The listing builds one solid part. Answer for the finished solid, in the listing's coordinates (mm). Face numbers are marked on the shaded views. A direction names the side the tool comes from. Round coordinates to 2 decimals unless told otherwise and drop trailing zeros. Write each loop counter-clockwise with the first axis right and the second up, starting at its lowest first coordinate (ties: lowest second). Pieces come first, ordered by that corner, then holes.
Item 1: Find section C-C on y = -3.75. Give the vertices of the cut face in (x, z).
Item 2: Each of these flat-tipped pins is pushed along its axis until it touches: pin 1 (3.5 mm diameter, centred on y = -4, z = -0.5, fed in from -X); pin 2 (1.2 mm diameter, centred on x = -0.5, y = -6.5, fed in from -Z); pin 3 (2.5 mm diameter, centred on x = -1.8, z = -1.2, fed in from -Y); pin 4 (1.5 mm diameter, centred on x = -1.5, z = 0.5, fed in from +Y). Where does it stop, or does it pass through?
Item 3: Find section A-A on x = 1.65. Give the vertices of the cut face in (y, z), then the cut area to 3 significant figures.
Item 4: A tool of negligible diameter and unlimited length cuts with its end or side. For the marked faces 5, 6 and 7, from which of +Z, -Z, +X, -X, +Y, -Y can it reach the whole face along a straight path? Write none if from no direction.
Item 5: Find section D-D on x = -0.55. Give the vertices of the cut face in (y, z), then the cut area to 3 significant figures.
Item 6: Find the intervals of material crossed by probe 1 along Y at (x, z) = (1.1, 0); probe 2 along X at (y, z) = (-7.05, 2.3); probe 3 along X at (y, z) = (-0.25, -2.25), in increasing order.
Item 7: For a pull along Z with two mould halves and no side action, classify the marked faces 1, 2, 3 and 4 as +Z half, -Z half, draft (parallel to the pull), parting line (faces both ways), or undercut.
Item 8: Find section B-B on z = 0. Give the vertices of the cut face in (x, y), then the cut area to 3 significant figures.
```python
from build123d import *

# Parameters (mm, degrees)
SKETCH_1_R          = 1.4
EXTRUDE_1_DEPTH     = 2
SKETCH_2_W          = 5.2
SKETCH_2_H          = 7
SKETCH_2_R          = 0.8
EXTRUDE_2_DEPTH     = 1.5
SKETCH_5_W          = 6
SKETCH_5_H          = 1
CUT_EXTRUDE_1_DEPTH = 2.5
CUT_EXTRUDE_2_REACH = 12.163
FILLET_1_R          = 0.2
FILLET_2_R          = 0.2
CHAMFER_1_SIZE      = 0.2


with BuildPart() as part:
    # 草图1 → 凸台-拉伸1 (new body)
    with BuildSketch(Plane(origin=(0, 0, 0), x_dir=(0, 0, -1), z_dir=(1, 0, 0))):
        with BuildLine():
            Line((3.5, 0), (3.5, -8))
            Line((3.5, -8), (-3.5, -8))
            Line((-3.5, -8), (-3.5, 0))
            ThreePointArc((-3.5, 0), (0, 3.5), (3.5, 0))
        make_face()
        Circle(SKETCH_1_R, mode=Mode.SUBTRACT)
    extrude(amount=EXTRUDE_1_DEPTH)

    # 草图2 → 凸台-拉伸2 (add)
    with BuildSketch(Plane.XZ.offset(8)):
        with Locations((-0.6, 0)):
            Rectangle(SKETCH_2_W, SKETCH_2_H)
        with Locations(Location((-1.8, -1.2, 0), (0, 0, 270))):
            Circle(SKETCH_2_R, mode=Mode.SUBTRACT)
        with Locations(Location((-1.8, 2.3, 0), (0, 0, 270))):
            Circle(SKETCH_2_R, mode=Mode.SUBTRACT)
    extrude(amount=-EXTRUDE_2_DEPTH)

    # 草图5 → 切除-拉伸1 (cut)
    with BuildSketch(Plane.XZ.offset(8)):
        with Locations((-1, -3)):
            Rectangle(SKETCH_5_W, SKETCH_5_H)
    extrude(amount=-CUT_EXTRUDE_1_DEPTH, mode=Mode.SUBTRACT)

    # 草图6 → 切除-拉伸2 (cut, up to next)
    with BuildSketch(Plane.ZY.offset(3.2), mode=Mode.PRIVATE) as cut_extrude_2_sk1:
        with BuildLine():
            Line((-1, -8.325127743), (-3.27705392, -8.325127743))
            Line((-3.27705392, -8.325127743), (-3.27705392, -6))
            Line((-3.27705392, -6), (-2.897366596, -6))
            ThreePointArc((-2.897366596, -6), (-2.378404875, -7.407669683), (-1, -8))
            Line((-1, -8), (-1, -8.325127743))
        make_face()
    cut_extrude_2_tool1 = extrude(cut_extrude_2_sk1.sketch, amount=-CUT_EXTRUDE_2_REACH, mode=Mode.PRIVATE) & part.part
    add(cut_extrude_2_tool1.solids().sort_by_distance((-3.2, -7.575754, -2.569334))[0], mode=Mode.SUBTRACT)

    # 圆角1
    fillet_1_edges = [part.edges().sort_by_distance(p)[0] for p in [
        (0, -6.5, 0.5),
    ]]
    fillet(fillet_1_edges, radius=FILLET_1_R)

    # 圆角2
    fillet_2_edges = [part.edges().sort_by_distance(p)[0] for p in [
        (2, 3.5, 0),
        (2, -4, 3.5),
        (-3.2, -8, 1.25),
        (-3.2, -6.5, 0.5),
        (0, -2.75, -3.5),
        (2, -2.75, -3.5),
        (0, -3.15, 3.5),
        (1, -5.5, -2.5),
        (0, -5.9, -2.5),
        (1, -5.5, -3.5),
        (0, 3.5, 0),
        (2, -5.5, -3),
        (2, -6.383095189, -2.5),
        (0, -5.5, -3),
        (-3.2, -7.806716397, -1.834936608),
        (-0.6, -7.266190379, -2.5),
        (-0.6, -8, 3.5),
        (-1.7, -6.5, -2.5),
        (-1.7, -6.5, 3.5),
        (-0.058578644, -6.441421356, -2.5),
        (-0.058578644, -6.441421356, 3.5),
    ]]
    fillet(fillet_2_edges, radius=FILLET_2_R)

    # 倒角1
    chamfer_1_edges = [part.edges().sort_by_distance(p)[0] for p in [
        (0, 0, 1.4),
        (2, 0, 1.4),
    ]]
    chamfer(chamfer_1_edges, length=CHAMFER_1_SIZE)


solid = part.part
```
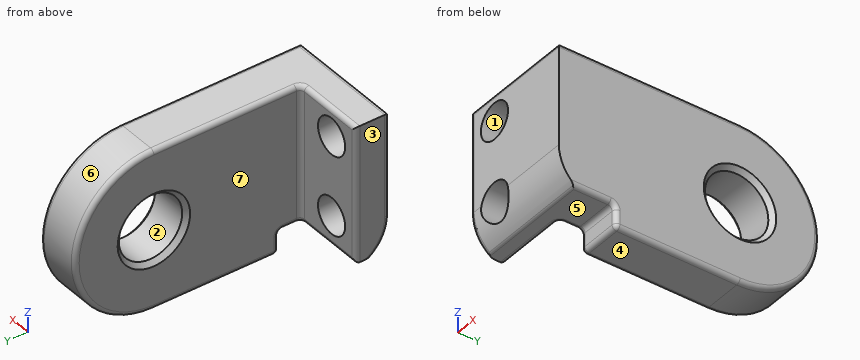
Check values:
1. outline: (0, -3.3) arc R0.2 ccw to (0.2, -3.5) - (1.8, -3.5) arc R0.2 ccw to (2, -3.3) - (2, 3.3) arc R0.2 ccw to (1.8, 3.5) - (0.2, 3.5) arc R0.2 ccw to (0, 3.3) - close
2. pin 1: stops at x = 0
2. pin 2: stops at z = -2.5
2. pin 3: stops at y = -8
2. pin 4: stops at y = -6.5
3. outline: (-8, -1) arc R1.9 ccw to (-7.32, -2.45) arc R0.2 ccw to (-7.2, -2.5) - (-5.7, -2.5) arc R0.2 cw to (-5.5, -2.7) - (-5.5, -3.3) arc R0.2 ccw to (-5.3, -3.5) - (0, -3.5) arc R3.5 ccw to (0, 3.5) - (-7.8, 3.5) arc R0.2 ccw to (-8, 3.3) - close; hole circle Ø2.8 at (0, 0)
3. area: 66.2 mm2
4. face 5: -Z, +X, -X, -Y
4. face 6: +X, -X, +Y
4. face 7: +Z, -Z, -X, +Y
5. outline: (-8, -1) arc R1.9 ccw to (-7.32, -2.45) arc R0.2 ccw to (-7.2, -2.5) - (-6.7, -2.5) arc R0.2 ccw to (-6.5, -2.3) - (-6.5, 3.3) arc R0.2 ccw to (-6.7, 3.5) - (-7.8, 3.5) arc R0.2 ccw to (-8, 3.3) - close
5. area: 8.64 mm2
6. probe 1: y = -8 to -1.4, 1.4 to 3.5
6. probe 2: x = -3.2 to -2.6, -1 to 2
6. probe 3: x = 0 to 2
7. face 1: undercut
7. face 2: undercut
7. face 3: draft
7. face 4: -Z half
8. outline: (-3.2, -7.8) arc R0.2 ccw to (-3, -8) - (2, -8) - (2, -1.6) - (1.8, -1.4) - (0.2, -1.4) - (0, -1.6) - (0, -6.3) arc R0.2 cw to (-0.2, -6.5) - (-3, -6.5) arc R0.2 ccw to (-3.2, -6.7) - close; (0, 1.6) - (0.2, 1.4) - (1.8, 1.4) - (2, 1.6) - (2, 3.3) arc R0.2 ccw to (1.8, 3.5) - (0.2, 3.5) arc R0.2 ccw to (0, 3.3) - close
8. area: 22.1 mm2
